Design review of the part built by this model. Coordinates are the model's own, in mm. Face numbers are marked on the shaded views. Coordinates: 2 decimals unless noted, no trailing zeros. Write each loop counter-clockwise with the first axis right and the second up, starting at its lowest first coordinate (ties: lowest second). Pieces come first, ordered by that corner, then holes.
Q1. The part is to be moulded in two halves that separate along X. For the marked faces 1, 2 and 3, say which applies: +X half, -X half, draft (parallel to the pull), parting line (faces both ways), or undercut.
Q2. Clearance check with flat-ended pins moving along their axes: pin 1 Ø7.5 at (x, y) = (-20.35, -4) entering from -Z; pin 2 Ø0.6 at (x, z) = (-26.5, 9) entering from +Y; pin 3 Ø0.6 at (y, z) = (-17.5, 8.5) entering from +X. State where each tip first meets the part, or that it passes through.
Q3. To check wall thickness, follow probe 1 along X at (y, z) = (2.5, 2); probe 2 along Y at (x, z) = (53.85, 4.3); probe 3 along Y at (x, z) = (-20.35, 5.4). State the ranges of each line that lie inside material, in increasing order.
Q4. Add section D-D, the plane y = -15. Give the boundary of the cut face in (x, z) (3 decimals), plus the area to 3 significant figures.
Q5. Add section C-C, the plane x = 5. Give the boundary of the cut face in (y, z).
Q6. Add section A-A, the plane x = 41. Give the boundary of the cut face in (y, z).
Q7. Add section B-B, the plane y = -4. Give the boundary of the cut face in (x, z), plus the area to 3 significant figures.
from build123d import *

# Parameters (mm, degrees)
F0_W      = 112.7
F0_H      = 36
F1_DEPTH  = 8
F3_W      = 54
F3_H      = 2
F4_DEPTH  = 2
F5_R      = 3.27
F6_DEPTH  = 8.001
F7_R      = 1.35
F8_DEPTH  = 5.5
F10_R     = 5.25
F11_DEPTH = 4.5
F9_W      = 20
F9_H      = 24
F9_W_2    = 27
F9_W_3    = 8.7
F9_H_2    = 8
F12_DEPTH = 10.001
F13_R     = 3.99999
F14_R     = 2.795
F15_DEPTH = 4.8
F16_R     = 2.795
F17_DEPTH = 4.8


# Not quite as in the source:
# - a fillet or chamfer is up to 0.001 mm smaller than in the source, because OpenCascade refuses the exact size


with BuildPart() as f1:
    # F0 (on Top) → F1 (new body)
    with BuildSketch(Plane.XY):
        Rectangle(F0_W, F0_H)
    extrude(amount=F1_DEPTH)

    # F3 (on face) → F4 (join)
    with BuildSketch(Plane.XY.offset(8)):
        with Locations((-19.35, -17)):
            Rectangle(F3_W, F3_H)
    extrude(amount=F4_DEPTH)

    # F5 (on face) → F6 (cut, through all)
    with BuildSketch(Plane.XY.offset(8)):
        with Locations((-20.35, -4)):
            Circle(F5_R)
    extrude(amount=-F6_DEPTH, mode=Mode.SUBTRACT)

    # F7 (on face) → F8 (cut)
    with BuildSketch(Plane(origin=(0, 0, 0), x_dir=(1, 0, 0), z_dir=(0, 0, -1))):
        with Locations((-53.85, 15)):
            Circle(F7_R)
        with Locations((-53.85, -15)):
            Circle(F7_R)
        with Locations((53.85, 15)):
            Circle(F7_R)
        with Locations((53.85, -15)):
            Circle(F7_R)
    extrude(amount=-F8_DEPTH, mode=Mode.SUBTRACT)

    # F10 (on face) → F11 (cut)
    with BuildSketch(Plane(origin=(0, 0, 0), x_dir=(1, 0, 0), z_dir=(0, 0, -1))):
        with Locations((-20.35, 4)):
            Circle(F10_R)
    extrude(amount=-F11_DEPTH, mode=Mode.SUBTRACT)

    # F9 (on face) → F12 (cut, through all)
    with BuildSketch(Plane(origin=(0, 0, 0), x_dir=(1, 0, 0), z_dir=(0, 0, -1))):
        with Locations((-40.35, 0)):
            Rectangle(F9_W, F9_H)
        with Locations((3.85, 0)):
            Rectangle(F9_W_2, F9_H)
        with Locations((36.85, 0)):
            Rectangle(F9_W_2, F9_H)
        with Locations((-20, -8)):
            Rectangle(F9_W_3, F9_H_2)
    extrude(amount=-F12_DEPTH, mode=Mode.SUBTRACT)

    # F13 (radius 4 in the source; OpenCascade refuses exactly that, so slightly less here)
    f13_edges = [f1.edges().sort_by_distance(p)[0] for p in [
        (-30.35, -12, 4),
        (-50.35, -12, 4),
        (-50.35, 12, 4),
        (-30.35, 12, 4),
        (-24.35, 4, 4),
        (-9.65, -12, 4),
        (23.35, -12, 4),
        (-9.65, 12, 4),
        (-24.35, 12, 4),
        (17.35, -12, 4),
        (50.35, -12, 4),
        (50.35, 12, 4),
        (23.35, 12, 4),
        (-15.65, 4, 4),
        (-15.65, 12, 4),
        (17.35, 12, 4),
    ]]
    fillet(f13_edges, radius=F13_R)

    # F14 (on face) → F15 (cut)
    with BuildSketch(Plane.XZ.offset(18)):
        with Locations((48.35, 4)):
            Circle(F14_R)
        with Locations((-48.35, 4)):
            Circle(F14_R)
    extrude(amount=-F15_DEPTH, mode=Mode.SUBTRACT)

    # F16 (on face) → F17 (cut)
    with BuildSketch(Plane(origin=(0, 18, 0), x_dir=(-1, 0, 0), z_dir=(0, 1, 0))):
        with Locations((48.35, 4)):
            Circle(F16_R)
        with Locations((-48.35, 4)):
            Circle(F16_R)
    extrude(amount=-F17_DEPTH, mode=Mode.SUBTRACT)


solid = f1.part
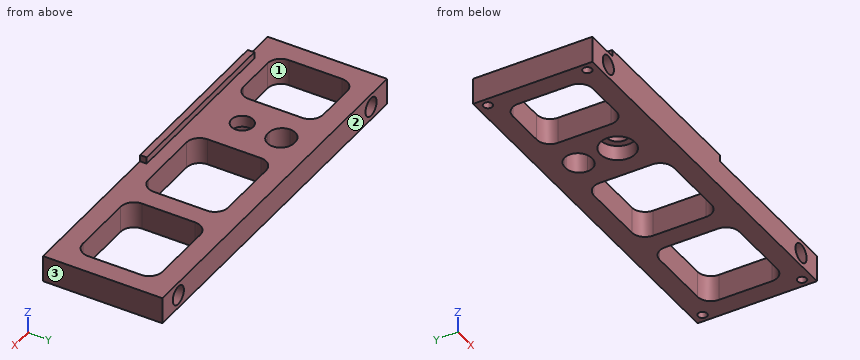
Here are the results:
1. face 1: undercut
1. face 2: draft
1. face 3: +X half
2. pin 1: stops at z = 4.5
2. pin 2: stops at y = -16
2. pin 3: stops at x = 7.65
3. probe 1: x = -56.35 to -50.35, -30.35 to -9.65, 17.35 to 23.35, 50.35 to 56.35
3. probe 2: y = -18 to -16.35, -13.65 to 13.65, 16.35 to 18
3. probe 3: y = -18 to -7.27, -0.73 to 4, 12 to 18
4. outline: (-56.35, 0) - (-55.2, 0) - (-55.2, 5.5) - (-52.5, 5.5) - (-52.5, 0) - (52.5, 0) - (52.5, 5.5) - (55.2, 5.5) - (55.2, 0) - (56.35, 0) - (56.35, 8) - (-56.35, 8) - close; hole circle Ø5.59 at (-48.35, 4); hole circle Ø5.59 at (48.35, 4)
4. area: 823 mm2
5. outline: (-18, 0) - (-12, 0) - (-12, 8) - (-16, 8) - (-16, 10) - (-18, 10) - close; (12, 0) - (18, 0) - (18, 8) - (12, 8) - close
6. outline: (-18, 0) - (-12, 0) - (-12, 8) - (-18, 8) - close; (12, 0) - (18, 0) - (18, 8) - (12, 8) - close
7. outline: (-56.35, 0) - (-50.35, 0) - (-50.35, 8) - (-56.35, 8) - close; (-30.35, 0) - (-25.6, 0) - (-25.6, 4.5) - (-23.62, 4.5) - (-23.62, 8) - (-30.35, 8) - close; (-17.08, 4.5) - (-15.1, 4.5) - (-15.1, 0) - (-9.65, 0) - (-9.65, 8) - (-17.08, 8) - close; (17.35, 0) - (23.35, 0) - (23.35, 8) - (17.35, 8) - close; (50.35, 0) - (56.35, 0) - (56.35, 8) - (50.35, 8) - close
7. area: 239 mm2
